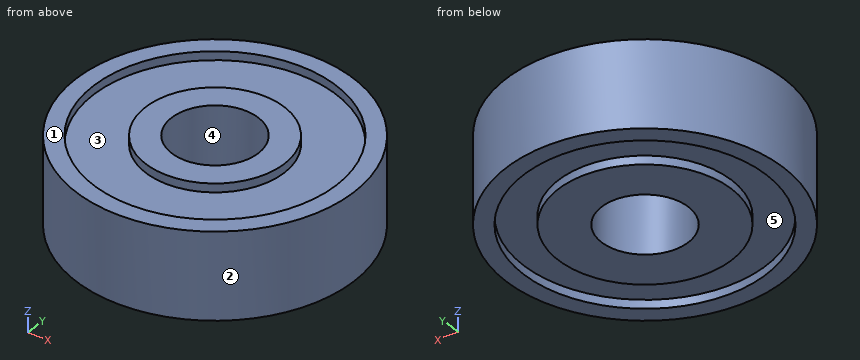
from build123d import *

# Parameters (mm, degrees)
ESQUISSE1_R             = 8
ESQUISSE1_R_2           = 7
BOSS_EXTRU_1_DEPTH      = 5
ESQUISSE1_3_R           = 7
ESQUISSE1_3_R_2         = 4
BOSS_EXTRU_2_DEPTH      = 4.5
ESQUISSE1_4_R           = 4
ESQUISSE1_4_R_2         = 2.5
BOSS_EXTRU_3_DEPTH      = 5
ESQUISSE2_R             = 7
ESQUISSE2_R_2           = 5
ENL_V_MAT_EXTRU_2_DEPTH = 0.5


with BuildPart() as part:
    # Esquisse1 → Boss.-Extru.1 (new body)
    with BuildSketch(Plane.XY):
        Circle(ESQUISSE1_R)
        Circle(ESQUISSE1_R_2, mode=Mode.SUBTRACT)
    extrude(amount=BOSS_EXTRU_1_DEPTH)

    # Esquisse1_3 → Boss.-Extru.2 (add)
    with BuildSketch(Plane.XY):
        Circle(ESQUISSE1_3_R)
        Circle(ESQUISSE1_3_R_2, mode=Mode.SUBTRACT)
    extrude(amount=BOSS_EXTRU_2_DEPTH)

    # Esquisse1_4 → Boss.-Extru.3 (add)
    with BuildSketch(Plane.XY):
        Circle(ESQUISSE1_4_R)
        Circle(ESQUISSE1_4_R_2, mode=Mode.SUBTRACT)
    extrude(amount=BOSS_EXTRU_3_DEPTH)

    # Esquisse2 → Enl_v. mat.-Extru.2 (cut)
    with BuildSketch(Plane(origin=(0, 0, 0), x_dir=(-1, 0, 0), z_dir=(0, 0, -1))):
        with Locations(Location((0, 0, 0), (0, 0, 180))):
            Circle(ESQUISSE2_R)
        Circle(ESQUISSE2_R_2, mode=Mode.SUBTRACT)
    extrude(amount=-ENL_V_MAT_EXTRU_2_DEPTH, mode=Mode.SUBTRACT)


solid = part.part
Verification items for the finished model (mm, model axes). Face numbers are marked on the shaded views. A direction names the side the tool comes from. Round coordinates to 2 decimals unless told otherwise and drop trailing zeros. Loops run counter-clockwise (first coordinate to the right, second up) from the corner with the lowest first, then second, coordinate; pieces in that order, holes last. Notation, with made-up numbers: (-32.5, -20) - (11.5, -20) arc R29 ccw to (11.5, 13) - close; hole circle Ø6 at (-1.5, -5.5). An arc over 180 degrees is marked (long way). Use a Markdown table: item, result. Add a question column.
1. Section check D-D, the plane y = 5.75. Record the boundary of the cut face in (x, z), plus the area to 3 significant figures.
2. Section check A-A, the plane x = 0. Record the boundary of the cut face in (y, z).
3. Section check C-C, the plane z = 1.25. Record the boundary of the cut face in (x, y), plus the area to 3 significant figures.
4. Release check for a two-part mould opening along Y. For the marked faces 1, 2 and 3 record: released by +Y, released by -Y, zero draft, split by the parting line, or undercut.
5. Gauge pin test, flat ends, axial feed: pin 1 (1 mm diameter, centred on x = -1, z = 4, fed in from +Y); pin 2 (1 mm diameter, centred on y = -5.5, z = 4, fed in from -X) (3 decimals). Record the tip position at first contact, or that the pin passes through.
6. Access from +Z, -Z, +X, -X, +Y, -Y to the whole of each face (thin tool, end or side, straight path). Record for the marked faces 4 and 5.
7. Thickness scan on probe 1 along Y at (x, z) = (0, 0.25); probe 2 along Y at (x, z) = (0, 4.85); probe 3 along Z at (x, y) = (4.25, 1). Record the ranges inside material, lowest first. Write a range as [from, to].
Checks:
| question | item | result |
|---|---|---|
| 1 | outline | (-5.56, 0) - (-3.99, 0) - (-3.99, 0.5) - (3.99, 0.5) - (3.99, 0) - (5.56, 0) - (5.56, 5) - (3.99, 5) - (3.99, 4.5) - (-3.99, 4.5) - (-3.99, 5) - (-5.56, 5) - close |
| 1 | area | 47.6 mm^2 |
| 2 | outline | (-8, 0) - (-7, 0) - (-7, 0.5) - (-5, 0.5) - (-5, 0) - (-2.5, 0) - (-2.5, 5) - (-4, 5) - (-4, 4.5) - (-7, 4.5) - (-7, 5) - (-8, 5) - close; (2.5, 0) - (5, 0) - (5, 0.5) - (7, 0.5) - (7, 0) - (8, 0) - (8, 5) - (7, 5) - (7, 4.5) - (4, 4.5) - (4, 5) - (2.5, 5) - close |
| 3 | outline | circle Ø16 at (0, 0); hole circle Ø5 at (0, 0) |
| 3 | area | 181 mm^2 |
| 4 | face 1 | zero draft |
| 4 | face 2 | split by the parting line |
| 4 | face 3 | undercut |
| 5 | pin 1 | stops at y = 7.98 |
| 5 | pin 2 | stops at x = -6.245 |
| 6 | face 4 | +Z, -Z |
| 6 | face 5 | -Z |
| 7 | probe 1 | y = [-8, -7], [-5, -2.5], [2.5, 5], [7, 8] |
| 7 | probe 2 | y = [-8, -7], [-4, -2.5], [2.5, 4], [7, 8] |
| 7 | probe 3 | z = [0, 4.5] |
